Can you work these out from the model? Positions are in its coordinate system, mm. Coordinates: 2 decimals unless noted, no trailing zeros. Loops run counter-clockwise (first coordinate to the right, second up) from the corner with the lowest first, then second, coordinate; pieces in that order, holes last. Notation, with made-up numbers: (61.25, 2) -> (100.25, 2) arc R28 cw to (100.25, 24) -> close; hole circle Ø3 at (22.25, 47.25). An arc over 180 degrees is marked (long way). Put each result on its own line as item: value. Start each with the question number.
Item 1: Will this pin go through, and if not, where does the flat tip stop? P1, Ø1.4, axis at x = -20.07, y = -116.17, coming from the -Z side.
Item 2: If we section it at C-C on z = 0.15: Please give me the cut outline in (x, y), plus the area to 3 significant figures.
Item 3: If we section it at A-A on x = -58.5: Please give me the cut outline in (y, z).
Item 4: If we section it at B-B on y = -52: Please give me the cut outline in (x, z).
Item 5: Please list where these lines run through material, in increasing order: L1, parallel to X at y = -5.5, z = 0.15; L2, parallel to Y at x = -23, z = 0.2; L3, parallel to Y at x = 53.5, z = 0.2. Write a range as from..to.
```python
from build123d import *

# Parameters (mm, degrees)
SKETCH1_R           = 114.3
SKETCH1_R_2         = 1.1303
SKETCH1_R_3         = 105
BOSS_EXTRUDE1_DEPTH = 0.254


with BuildPart() as part:
    # Sketch1 → Boss-Extrude1 (new body)
    with BuildSketch(Plane.XY):
        with Locations((-20.073709177, -8.103148659)):
            Circle(SKETCH1_R)
        with Locations((-113.658579374, -62.134398659)):
            Circle(SKETCH1_R_2, mode=Mode.SUBTRACT)
        with Locations((-20.073709177, -116.165648659)):
            Circle(SKETCH1_R_2, mode=Mode.SUBTRACT)
        with Locations((73.511161019, -62.134398659)):
            Circle(SKETCH1_R_2, mode=Mode.SUBTRACT)
        with Locations((73.511161019, 45.928101341)):
            Circle(SKETCH1_R_2, mode=Mode.SUBTRACT)
        with Locations((-20.073709177, 99.959351341)):
            Circle(SKETCH1_R_2, mode=Mode.SUBTRACT)
        with Locations((-20.073709177, -8.103148659)):
            Circle(SKETCH1_R_3, mode=Mode.SUBTRACT)
        with Locations((-113.658579374, 45.928101341)):
            Circle(SKETCH1_R_2, mode=Mode.SUBTRACT)
    extrude(amount=BOSS_EXTRUDE1_DEPTH)


solid = part.part
```
Solutions:
1. P1: through
2. outline: circle Ø228.6 at (-20.07, -8.1); hole circle Ø210 at (-20.07, -8.1); hole circle Ø2.26 at (-113.66, -62.13); hole circle Ø2.26 at (-113.66, 45.93); hole circle Ø2.26 at (-20.07, -116.17); hole circle Ø2.26 at (-20.07, 99.96); hole circle Ø2.26 at (73.51, -62.13); hole circle Ø2.26 at (73.51, 45.93)
2. area: 6,380 mm^2
3. outline: (-115.75, 0) -> (-105.82, 0) -> (-105.82, 0.25) -> (-115.75, 0.25) -> close; (89.61, 0) -> (99.54, 0) -> (99.54, 0.25) -> (89.61, 0.25) -> close
4. outline: (-125.61, 0) -> (-115.46, 0) -> (-115.46, 0.25) -> (-125.61, 0.25) -> close; (75.31, 0) -> (85.46, 0) -> (85.46, 0.25) -> (75.31, 0.25) -> close
5. L1: -134.34..-125.04, 84.89..94.2
5. L2: -122.37..-113.06, 96.86..106.16
5. L3: -95.58..-83.02, 66.81..79.37
